CAD build for the part. Positions are in the model's coordinates, mm. A direction names the side the tool comes from. Round coordinates to 2 decimals unless told otherwise and drop trailing zeros. Loops run counter-clockwise (first coordinate to the right, second up) from the corner with the lowest first, then second, coordinate; pieces in that order, holes last.
Autodesk Inventor part; units mm, degrees
ref_plane "YZ Plane" through (0, 0, 0) normal (1, 0, 0) x (0, 1, 0)
ref_plane "XZ Plane" through (0, 0, 0) normal (0, 1, 0) x (-1, 0, 0)
ref_plane "XY Plane" through (0, 0, 0) normal (0, 0, 1) x (1, 0, 0)
sketch "Sketch1" plane through (0, 0, 0) normal (0, 1, 0) x (-1, 0, 0)
  line L0 (2, -7) -> (2, 2)
  line L1 (2, 2) -> (0, 2)
  arc A0 (0, 2) -> (0, -2) centre (0, 0) ccw
  line L2 (0, -2) -> (0, -7)
  line L3 (0, -7) -> (2, -7)
  circle A1 centre (0, 0) radius 0.35
  dimension "d0" = 5
  dimension "d1" = 2
  dimension "d2" = 2
  dimension "d3" = 0.7
extrude "Extrusion1" add sketch "Sketch1" along normal mid plane 12
sketch "Sketch2" plane through (0, -6, -7) normal (1, 0, 0) x (0, 0, -1)
  line L0 (0, 12) -> (0, 0)
  line L1 (-5, 12) -> (0, 12)
  line L2 (-5, 12) -> (-5, 0)
  line L3 (0, 0) -> (-5, 0)
  circle A0 centre (-2.5, 2.5) radius 2.5 construction
  line L4 (0, 0) -> (-5, 0) construction
  circle A1 centre (-2.5, 9.5) radius 2.5 construction
  line L5 (0, 12) -> (-9, 12) construction
  line L6 (-5, 12) -> (-5, 0) construction
  line L7 (0, 12) -> (0, 0) construction
  point P0 (-7, 6)
hole "Hole1" at (0, -3.5, -4.5) at (0, 3.5, -4.5) direction (-1, 0, 0) diameter 3 end through all
sketch "Sketch3" plane through (0, -6, -7) normal (1, 0, 0) x (0, 0, -1)
  circle A0 centre (-2.5, 2.5) radius 1.5
  circle A1 centre (-2.5, 9.5) radius 1.5
  line L0 (0, 12) -> (0, 0)
  line L1 (-5, 12) -> (0, 12)
  line L2 (-5, 12) -> (-5, 0)
  line L3 (0, 0) -> (-5, 0)
  line L4 (-9, 3.5) -> (-6, 3.5)
  line L5 (-5, 4.5) -> (-5, 7.5)
  line L6 (-6, 8.5) -> (-9, 8.5)
  line L7 (-9, 8.5) -> (-9, 3.5)
  arc A2 (-6, 3.5) -> (-5, 4.5) centre (-6, 4.5) ccw
  arc A3 (-5, 7.5) -> (-6, 8.5) centre (-6, 7.5) ccw
  line L8 (-9, 0) -> (-9, 12)
  point P0 (-7, 6)
  point P1 (-9, 6)
  dimension "d13" = 1
  dimension "d14" = 5
extrude "Extrusion2" cut sketch "Sketch3" along normal through all both and the other way through all contours L2 A2 L4 L7 L6 A3
sketch "Sketch4" plane through (0, -6, 0) normal (0, -1, 0) x (1, 0, 0)
  circle A0 centre (0, 0) radius 0.35
  line L0 (-2, 2) -> (-2, -7)
  line L1 (-2, -7) -> (0, -7)
  line L2 (0, -7) -> (0, -2)
  arc A1 (0, -2) -> (0, 2) centre (0, 0) ccw
  line L3 (0, 2) -> (-2, 2)
  arc A2 (0, -2) -> (0, 2) centre (0, 0) ccw
  line L4 (0, -7) -> (0, -2)
  line L5 (0, -2) -> (-2, -2)
  line L6 (-2, 2) -> (-2, -7)
extrude "Extrusion3" add sketch "Sketch4" along normal blind 10 contours L3 A1 L5 L0
sketch "Sketch5" plane through (-2, -6, -7) normal (-1, 0, 0) x (0, 0, 1)
  line L0 (9, 3.5) -> (6, 3.5)
  arc A0 (5, 4.5) -> (6, 3.5) centre (6, 4.5) ccw
  line L1 (5, 4.5) -> (5, 7.5)
  arc A1 (6, 8.5) -> (5, 7.5) centre (6, 7.5) ccw
  line L2 (6, 8.5) -> (9, 8.5)
  line L3 (9, 8.5) -> (9, 12)
  line L4 (0, 12) -> (9, 12)
  line L5 (0, 12) -> (0, 0)
  line L6 (5, 0) -> (0, 0)
  line L7 (5, 0) -> (5, -10)
  line L8 (9, -10) -> (5, -10)
  line L9 (9, -10) -> (9, 3.5)
  circle A2 centre (2.5, 9.5) radius 1.5
  circle A3 centre (2.5, 2.5) radius 1.5
  arc A4 (7.35, -1) -> (6.35, 0) centre (6.35, -1) ccw
  line L10 (9, 3.5) -> (9, -10)
  arc A5 (7.35, -1) -> (9, -5.5141) centre (14.35, -1) ccw
  line L11 (5, 4.5) -> (5, 0)
  line L12 (5, 0) -> (6.35, 0)
  line L13 (7.35, -10) -> (6.65, -10) construction
  line L14 (6, 3.5) -> (9, 3.5) construction
  line L15 (9, -10) -> (9, 3.5) construction
  line L16 (9, -5.5141) -> (9, -10)
  line L17 (7.35, -10) -> (7.35, 3.5)
  arc A6 (8.5426, -4.9082) -> (9, -4.7686) centre (8.75, -4.7686) ccw
  line L18 (9, -5.5141) -> (9, -4.7686)
  point P0 (7, 6)
  dimension "d19" = 7
  dimension "d22" = 0.25
  dimension "d23" = 33.939
extrude "Extrusion4" cut sketch "Sketch5" against normal through all contours L9 A5 A6 | L17 L8 L7 L12 A4 | A5 L9 L8 L17
mirror "Mirror1" about plane through (0, 0, 0) normal (0, 1, 0) of "Extrusion3", "Extrusion4"
properties part number "+XPanel_AntennaMount" material "Acetal Resin, Black"
Item 1: Cut at C-C, the plane z = -4.5. Give the cut face in (x, y), plus the area to 3 significant figures.
Answers follow:
outline: (-2, -6) - (0, -6) - (0, -5) - (-2, -5) - close; (-2, -2) - (0, -2) - (0, 2) - (-2, 2) - close; (-2, 5) - (0, 5) - (0, 6) - (-2, 6) - close
area: 12.0 mm2
Item 2: Cut at D-D, the plane z = 0. Give the cut face in (x, y).
Answers follow:
outline: (-2, -6.24) - (-0.35, -6.24) - (-0.35, -2.5) - (-2, -2.5) - close; (-2, 2.5) - (-0.35, 2.5) - (-0.35, 6.24) - (-2, 6.24) - close; (0.35, -6.24) - (2, -6.24) - (2, -2.5) - (0.35, -2.5) - close; (0.35, 2.5) - (2, 2.5) - (2, 6.24) - (0.35, 6.24) - close
Item 3: Two-plate mould, pull along Z, no slides. Class faces 4 (the cylindrical face through (-1.014, -2.925, -5.886)), 5 (the flat face through (-1, -7, 2)), 6 (the cylindrical face through (-0.043, 9.071, 0.663)): released by +Z, released by -Z, zero draft, split by the parting line, or undercut.
Answers follow:
face 4: undercut
face 5: released by +Z
face 6: released by -Z
Item 4: Cut at A-A, the plane y = -3.5. Give the cut face in (x, z).
Answers follow:
outline: (-2, -7) - (0, -7) - (0, -6) - (-2, -6) - close; (-2, -3) - (0, -3) - (0, -2) arc R2 ccw to (0, 2) - (-2, 2) - close; hole circle Ø0.7 at (0, 0)
Item 5: Cut at B-B, the plane x = -1.65. Give the cut face in (y, z).
Answers follow:
outline: (-10.91, 1.54) arc R7 ccw to (-7, 0.35) arc R1 cw to (-6, -0.65) - (-6, -7) - (6, -7) - (6, -0.65) arc R1 cw to (7, 0.35) arc R7 ccw to (10.91, 1.54) arc R0.25 ccw to (10.77, 2) - (2.5, 2) - (2.5, -1) arc R1 cw to (1.5, -2) - (-1.5, -2) arc R1 cw to (-2.5, -1) - (-2.5, 2) - (-10.77, 2) arc R0.25 ccw to start; hole circle Ø3 at (-3.5, -4.5); hole circle Ø3 at (3.5, -4.5)
Item 6: Flat gauge pins, fed straight in: P1, Ø1.2, axis at x = 0, z = -3.5, coming from the -Y side; P2, Ø0.6, axis at x = -1.5, y = 0.5, coming from the +Z side; P3, Ø1, axis at y = -2.5, z = -1, coming from the +X side. Where does each tip first touch, or does it go through?
Answers follow:
P1: stops at y = -6
P2: stops at z = -2
P3: stops at x = 1.94
Item 7: Probe line 1 (Y direction, x = -0.8, z = -4.5); line 2 (X direction, y = -3.35, z = 0); line 3 (Y direction, x = -0.5, z = -3.5). List the from-to ranges inside material, lowest first.
Answers follow:
line 1: y = -6 to -5, -2 to 2, 5 to 6
line 2: x = -2 to -0.35, 0.35 to 2
line 3: y = -6 to -4.62, -2.38 to 2.38, 4.62 to 6
Item 8: 3-axis set-ups, long thin cutter, end or side, ignore diameter. For faces 1 (the flat face through (0, 0, -4)), 2 (the flat face through (-1, 6, -4)), 3 (the cylindrical face through (-0.575, 2.215, -1.699)): which of +Z, -Z, +X, -X, +Y, -Y reach the whole face in a straight line?
Answers follow:
face 1: -Z, +X, +Y, -Y
face 2: -Z, +X, -X, +Y
face 3: +Z, +X, -X
